Design review of the part shown in the three views and the two pictorial views. Dimensions are in mm from the part's minimum x, y and z. A direction names the side the tool comes from. Give positions to 0.01 mm unless a question says otherwise; leave off trailing zeros. Loops run counter-clockwise (first coordinate to the right, second up) from the corner with the lowest first, then second, coordinate; pieces in that order, holes last. Notation, with made-up numbers: (10.25, -20) -> (67.25, -20) arc R33 ccw to (67.25, 11) -> close; hole circle Ø2 at (85, 51.5). An arc over 180 degrees is marked (long way). Answer as CSV lines item,"result".
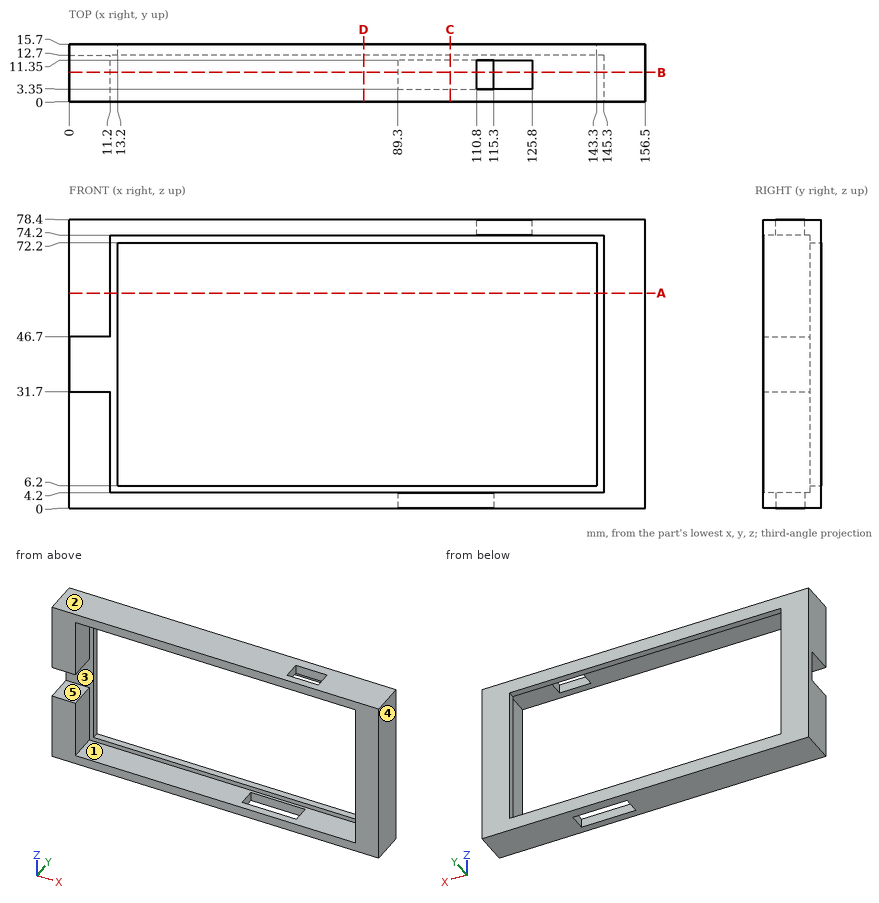
Q1. We need section C-C, the plane x = 103.5. State the section outline as (y, z) points.
Filled sheet:
outline,"(0, 0) -> (3.35, 0) -> (3.35, 4.2) -> (0, 4.2) -> close; (0, 74.2) -> (12.7, 74.2) -> (12.7, 72.2) -> (15.7, 72.2) -> (15.7, 78.4) -> (0, 78.4) -> close; (11.35, 0) -> (15.7, 0) -> (15.7, 6.2) -> (12.7, 6.2) -> (12.7, 4.2) -> (11.35, 4.2) -> close"
Q2. We need section A-A, the plane z = 58.5. State the section outline as (x, y) points, and give its area (3 significant figures).
Filled sheet:
outline,"(0, 0) -> (11.2, 0) -> (11.2, 12.7) -> (13.2, 12.7) -> (13.2, 15.7) -> (0, 15.7) -> close; (143.3, 12.7) -> (145.3, 12.7) -> (145.3, 0) -> (156.5, 0) -> (156.5, 15.7) -> (143.3, 15.7) -> close"
area,"364 mm^2"
Q3. The part is to be moulded in two halves that separate along X. For the marked faces 3, 4 and 5, say which applies: pulls with the +X half, pulls with the -X half, needs draft (parallel to the pull), parting line crosses it, or undercut.
Filled sheet:
face 3,"undercut"
face 4,"pulls with the +X half"
face 5,"needs draft"
Q4. To check wall thickness, follow probe 1 along X at (y, z) = (13.25, 10.5); probe 2 along X at (y, z) = (12.5, 17); probe 3 along Z at (x, y) = (53, 2.5). State the ranges of each line that lie inside material, in increasing order. Write a range as from..to.
Filled sheet:
probe 1,"x = 0..13.2, 143.3..156.5"
probe 2,"x = 0..11.2, 145.3..156.5"
probe 3,"z = 0..4.2, 74.2..78.4"
Q5. We need section D-D, the plane x = 80. State the section outline as (y, z) points.
Filled sheet:
outline,"(0, 0) -> (15.7, 0) -> (15.7, 6.2) -> (12.7, 6.2) -> (12.7, 4.2) -> (0, 4.2) -> close; (0, 74.2) -> (12.7, 74.2) -> (12.7, 72.2) -> (15.7, 72.2) -> (15.7, 78.4) -> (0, 78.4) -> close"
Q6. Clearance check with flat-ended pins moving along their axes: pin 1 Ø4.5 at (x, z) = (120.5, 76.5) entering from -Y; pin 2 Ø1 at (y, z) = (7.5, 41.5) entering from -X. State where each tip first meets the part, or that it passes through.
Filled sheet:
pin 1,"stops at y = 0"
pin 2,"stops at x = 145.3"
Q7. For the marked faces 1 and 2, list the 3-axis set-ups (+Z, -Z, +X, -X, +Y, -Y) from which the entire face can be reached by the end or side of a thin tool; tool diameter is ignored.
Filled sheet:
face 1,"-Y"
face 2,"+Z, +X, -X, +Y, -Y"
Q8. We need section B-B, the plane y = 8. State the section outline as (x, z) points.
Filled sheet:
outline,"(0, 0) -> (89.3, 0) -> (89.3, 4.2) -> (11.2, 4.2) -> (11.2, 31.7) -> (0, 31.7) -> close; (0, 46.7) -> (11.2, 46.7) -> (11.2, 74.2) -> (110.8, 74.2) -> (110.8, 78.4) -> (0, 78.4) -> close; (115.3, 0) -> (156.5, 0) -> (156.5, 78.4) -> (125.8, 78.4) -> (125.8, 74.2) -> (145.3, 74.2) -> (145.3, 4.2) -> (115.3, 4.2) -> close"
